from build123d import *

# Parameters (mm, degrees)
SKETCH_R     = 15
PAD_DEPTH    = 4
SKETCH001_R  = 13
PAD001_DEPTH = 5
FILLET_R     = 1


with BuildPart() as part:
    # Sketch → Pad (new body)
    with BuildSketch(Plane.XY):
        Circle(SKETCH_R)
    extrude(amount=PAD_DEPTH)

    # Sketch001 (on Face3 of Pad) → Pad001 (join)
    with BuildSketch(Plane.XY.offset(4)):
        Circle(SKETCH001_R)
    extrude(amount=PAD001_DEPTH)

    # Fillet
    fillet_edges = [part.edges().sort_by_distance(p)[0] for p in [
        (-13, 0, 9),
    ]]
    fillet(fillet_edges, radius=FILLET_R)


solid = part.part
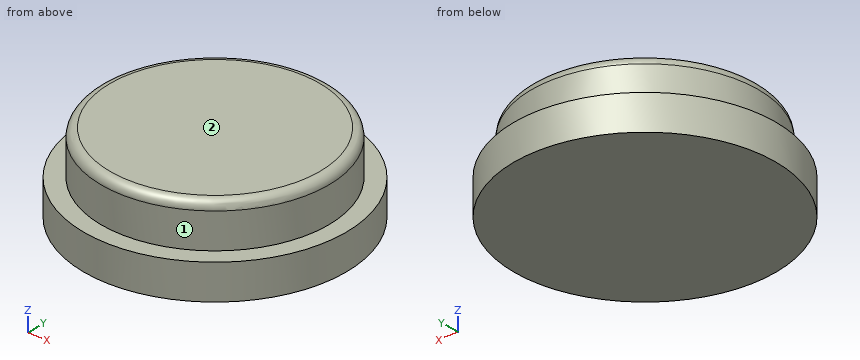
Can you work these out from the model? Positions are in its coordinate system, mm. Face numbers are marked on the shaded views. A direction names the side the tool comes from. Give positions to 0.01 mm unless a question says otherwise; leave off trailing zeros. Loops run counter-clockwise (first coordinate to the right, second up) from the corner with the lowest first, then second, coordinate; pieces in that order, holes last. Notation, with made-up numbers: M 82.25,2 L 99.25,2 A17 ccw 99.25,31 Z; hole C 82.5,50.25 d7. An arc over 180 degrees is marked long. One line per item, written item: value.
1) I'm going to push flat-ended pins straight in: pin 1 (4 mm diameter, centred on x = 4.5, z = 4.5, fed in from +Y); pin 2 (5 mm diameter, centred on x = -3.5, y = 9.5, fed in from -Z); pin 3 (2 mm diameter, centred on x = 4, z = 7, fed in from +Y); pin 4 (1 mm diameter, centred on y = 4.5, z = 2, fed in from +X). Where does each tip first touch, or does it pass through?
Geometry check:
pin 1: stops at y = 14.78
pin 2: stops at z = 0
pin 3: stops at y = 12.65
pin 4: stops at x = 14.46
2) Imagine slicing it at A-A on x = 0. Write out the boundary of the cut face in (y, z).
Geometry check:
outline: M -15,0 L 15,0 L 15,4 L 13,4 L 13,8 A1 ccw 12,9 L -12,9 A1 ccw -13,8 L -13,4 L -15,4 Z
3) Please list where these lines run through material, in increasing order: line 1 (Z direction, x = -11.5, y = 8.75); line 2 (X direction, y = 5, z = 5.25).
Geometry check:
line 1: z = 0 to 4
line 2: x = -12 to 12
4) On a 3-axis mill with a long thin cutter (end or side, diameter ignored), from which of +Z, -Z, +X, -X, +Y, -Y can I reach the whole of each face in a straight line? I mean the marked faces 1 and 2. Say none if no direction works.
Geometry check:
face 1: +Z
face 2: +Z, +X, -X, +Y, -Y
